Autodesk Inventor part; units mm, degrees
ref_plane "YZ Plane" through (0, 0, 0) normal (1, 0, 0) x (0, 1, 0)
ref_plane "XZ Plane" through (0, 0, 0) normal (0, 1, 0) x (-1, 0, 0)
ref_plane "XY Plane" through (0, 0, 0) normal (0, 0, 1) x (1, 0, 0)
sketch "Sketch1" plane through (0, 0, 0) normal (0, 1, 0) x (-1, 0, 0)
  line L0 (0.1032, -6.0991) -> (-407.6831, -12.9981)
  line L1 (0.1032, 6.0991) -> (-407.6831, 12.9981)
  arc A0 (0.1032, -6.0991) -> (0.1032, 6.0991) centre (0, 0) ccw
  arc A1 (-407.6831, 12.9981) -> (-407.6831, -12.9981) centre (-407.903, 0) ccw
  line L2 (-407.6598, 14.3779) -> (0.1265, 7.4789)
  arc A2 (0.1265, -7.4789) -> (0.1265, 7.4789) centre (0, 0) ccw
  line L3 (0.1265, -7.4789) -> (-407.6598, -14.3779)
  arc A3 (-407.6598, 14.3779) -> (-407.6598, -14.3779) centre (-407.903, 0) ccw
  dimension "d2" = 6.1
  dimension "d3" = 13
  dimension "d4" = 1.38
  dimension "d5" = 407.903
extrude "Extrusion1" add sketch "Sketch1" along normal blind 6
chamfer "Chamfer1" distance 0.2 angle 45 16 edges at (203.79, 6, 9.5486) (-6.1, 6, 0) (203.79, 6, -9.5486) (420.903, 6, 0) (203.7666, 6, 10.9284) (422.283, 6, 0) (203.7666, 6, -10.9284) (-7.48, 6, 0) (203.7666, 0, 10.9284) (-7.48, 0, 0) (203.7666, 0, -10.9284) (422.283, 0, 0) (203.79, 0, 9.5486) (420.903, 0, 0) (203.79, 0, -9.5486) (-6.1, 0, 0)
properties part number "y_axis_belt" material "Rubber"
Here's how the part is built. I have some questions about the finished solid (model axes, mm). Round coordinates to 2 decimals unless told otherwise and drop trailing zeros. Write each loop counter-clockwise with the first axis right and the second up, starting at its lowest first coordinate (ties: lowest second). Pieces come first, ordered by that corner, then holes.
Q1. If we mould it in two halves opening along X, with no side actions, what happens to faces 1 (the cylindrical face through (420.9, 3, -0.3)), 2 (the flat face through (208, 0, -10))? For each: +X half, -X half, draft (parallel to the pull), parting line (faces both ways), or undercut.
Q2. Will these pins go through, and if not, where does the flat tip stop? P1, Ø5, axis at x = 245, z = 6, coming from the -Y side; P2, Ø1, axis at x = 132, y = 1.5, coming from the +Z side; P3, Ø1.5, axis at y = 3.5, z = 11, coming from the +X side; P4, Ø1, axis at x = 38.5, y = 2.5, coming from the -Z side.
Q3. If we section it at C-C on x = 350: Write out the boundary of the cut face in (y, z), plus the area to 3 significant figures.
Q4. If we section it at B-B on y = 3.9: Write out the boundary of the cut face in (x, z).
Q5. If we section it at A-A on z = 0: Write out the boundary of the cut face in (x, y).
Q6. Please list where these lines run through material, in increasing order: probe 1 along X at (y, z) = (0.75, -0.25); probe 2 along X at (y, z) = (0.95, 1); probe 3 along Z at (x, y) = (34, 0.3).
Answer below:
1. face 1: undercut
1. face 2: draft
2. P1: passes through
2. P2: stops at z = 9.72
2. P3: stops at x = 417.99
2. P4: stops at z = -8.14
3. outline: (0, -13.2) - (0.2, -13.4) - (5.8, -13.4) - (6, -13.2) - (6, -12.22) - (5.8, -12.02) - (0.2, -12.02) - (0, -12.22) - close; (0, 12.22) - (0.2, 12.02) - (5.8, 12.02) - (6, 12.22) - (6, 13.2) - (5.8, 13.4) - (0.2, 13.4) - (0, 13.2) - close
3. area: 16.4 mm2
4. outline: (-0.13, -7.48) - (407.66, -14.38) arc R14.38 ccw (long way) to (407.66, 14.38) - (-0.13, 7.48) arc R7.48 ccw to start; hole (-0.1, -6.1) - (407.68, -13) arc R13 ccw (long way) to (407.68, 13) - (-0.1, 6.1) arc R6.1 ccw to start
5. outline: (-7.48, 0.2) - (-7.28, 0) - (-6.3, 0) - (-6.1, 0.2) - (-6.1, 5.8) - (-6.3, 6) - (-7.28, 6) - (-7.48, 5.8) - close; (420.9, 0.2) - (421.1, 0) - (422.08, 0) - (422.28, 0.2) - (422.28, 5.8) - (422.08, 6) - (421.1, 6) - (420.9, 5.8) - close
6. probe 1: x = -7.48 to -6.09, 420.9 to 422.28
6. probe 2: x = -7.41 to -6.02, 420.86 to 422.25
6. probe 3: z = -8.06 to -6.68, 6.68 to 8.06
